Could you check a few things on this model? Use its own coordinates, in mm. Give positions to 0.01 mm unless a question says otherwise; leave off trailing zeros. Order: outer loops, then holes, each group sorted by start corner. A loop starts at its lowest first (then second) coordinate and runs counter-clockwise, first axis right, second up. Notation, with made-up numbers: (-9.75, 87) -> (22.25, 87) arc R13 cw to (22.25, 112) -> close; hole circle Ø5 at (7, 11.25). An arc over 180 degrees is marked (long way). One line per item, written item: value.
```python
from build123d import *

# Parameters (mm, degrees)
F0_W     = 127
F0_H     = 127
F1_DEPTH = 133.096
F2_R     = 95.0475879506
F3_R     = 94.4343777058


with BuildPart() as f1:
    # F0 (on Right) → F1 (new body)
    with BuildSketch(Plane.YZ):
        with Locations((63.5, 63.5)):
            Rectangle(F0_W, F0_H)
    extrude(amount=F1_DEPTH)

    # F2
    f2_edges = [f1.edges().sort_by_distance(p)[0] for p in [
        (133.096, 63.5, 127),
    ]]
    fillet(f2_edges, radius=F2_R)

    # F3
    f3_edges = [f1.edges().sort_by_distance(p)[0] for p in [
        (105.257206, 0, 99.161206),
    ]]
    fillet(f3_edges, radius=F3_R)


solid = f1.part
```
1) Suppose I cut it at A-A, the plane z = 13.5. Write out the boundary of the cut face in (x, y), then the cut area to 3 significant figures.
Answer below:
outline: (0, 0) -> (38.66, 0) arc R94.43 ccw to (133.1, 94.43) -> (133.1, 127) -> (0, 127) -> close
area: 15,000 mm2
2) For P1, Ø4, axis at y = 104.5, z = 89, coming from the +X side; P2, Ø3, axis at x = 62, z = 104, coming from the -Y side; P3, Ø1.5, axis at x = 67, y = 80, coming from the +Z side, each with a flat end and sliding along its axis, tell me the tip position at first contact or that it passes through.
Answer below:
P1: stops at x = 115.53
P2: stops at y = 35.53
P3: stops at z = 121.59
3) If I drill on line 1 along X through (y, z) = (92, 14); line 2 along Z through (x, y) = (79.5, 78.5); line 3 along Y through (x, z) = (40, 98), over which ranges is the centre line in solid material (lowest first)?
Answer below:
line 1: x = 0 to 133.06
line 2: z = 0 to 115.98
line 3: y = 26.37 to 127
4) Suppose I cut it at B-B, the plane x = 30.5. Write out the boundary of the cut face in (y, z), then the cut area to 3 significant figures.
Answer below:
outline: (0, 0) -> (127, 0) -> (127, 127) -> (94.43, 127) arc R94.43 ccw to (0, 32.57) -> close
area: 14,200 mm2
